The listing builds one solid part. Answer for the finished solid, in the listing's coordinates (mm). Give positions to 0.01 mm unless a question says otherwise; leave off trailing zeros. Write each loop counter-clockwise with the first axis right and the second up, starting at its lowest first coordinate (ties: lowest second). Pieces come first, ordered by that corner, then holes. Notation, with made-up numbers: M 87.5,28 L 124.5,28 A32 ccw 124.5,64 Z; hole C 39,-39.75 d10. An arc over 180 degrees is marked long. Return JSON: item names as keys, results as strings.
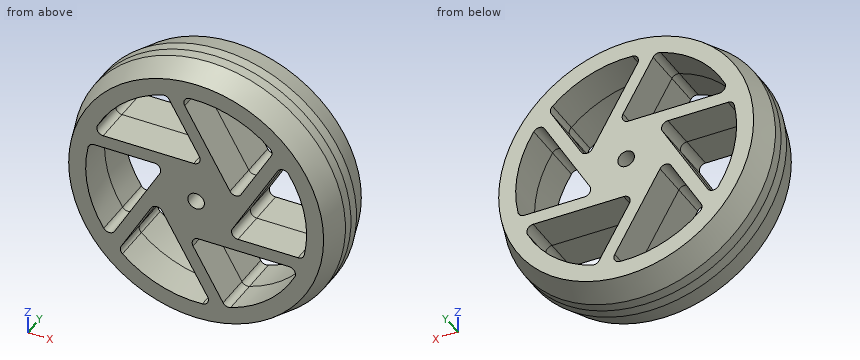
from build123d import *

# Parameters (mm, degrees)
CUT_EXTRUDE1_REACH             = 48.046
CUT_EXTRUDE1_DIRECTION_2_REACH = 48.046
CIRPATTERN1_COUNT              = 6
CUT_EXTRUDE2_DEPTH             = 15
CUT_EXTRUDE2_DEPTH_BACK        = 15
SKETCH6_R                      = 1.95


with BuildPart() as part:
    # Sketch2 → Revolve1 (revolve)
    with BuildSketch(Plane.XY, mode=Mode.PRIVATE) as revolve1_sk:
        Polygon((0, 0), (32, 0), (32, 2.5), (30, 8.5), (0, 8.5), align=None)
    revolve1 = revolve(revolve1_sk.sketch.rotate(Axis((0, 8.5, 0), (0, -1, 0)), 90), axis=Axis((0, 8.5, 0), (0, -1, 0)))

    # Mirror1: Revolve1 across plane
    add(revolve1.mirror(Plane.ZX))

    # Cut-Extrude1: up to this face of the body (flat: up to its plane)
    cut_extrude1_end = Plane(part.part.faces().sort_by_distance((0, 8.5, 0))[0])
    # Sketch3 → Cut-Extrude1 (cut, up to the picked face)
    with BuildSketch(Plane(origin=(0, 0, 0), x_dir=(1, 0, 0), z_dir=(0, 1, 0)), mode=Mode.PRIVATE) as cut_extrude1_sk1:
        with BuildLine():
            Line((0.562177826, 9.526279442), (5.5, 9.526279442))
            Line((5.5, 9.526279442), (21.878554835, 9.526279442))
            ThreePointArc((21.878554835, 9.526279442), (23.155781812, 10.23971015), (23.218058192, 11.701357775))
            ThreePointArc((23.218058192, 11.701357775), (16.957041557, 19.709356703), (8.104096566, 24.704728674))
            ThreePointArc((8.104096566, 24.704728674), (7.100974397, 24.680582577), (6.337514428, 24.029455866))
            Line((6.337514428, 24.029455866), (-0.736860279, 11.776279442))
            ThreePointArc((-0.736860279, 11.776279442), (-0.736860279, 10.276279442), (0.562177826, 9.526279442))
        make_face()
    cut_extrude1_tool1 = split(extrude(cut_extrude1_sk1.sketch, amount=CUT_EXTRUDE1_REACH, mode=Mode.PRIVATE), bisect_by=cut_extrude1_end, keep=Keep.BOTH, mode=Mode.PRIVATE)
    cut_extrude1 = cut_extrude1_tool1.solids().sort_by(Axis((10.856856, 0, -15.344995), (0, 1, 0)))[0]
    add(cut_extrude1, mode=Mode.SUBTRACT)

    # Cut-Extrude1 direction 2: up to this face of the body (flat: up to its plane)
    cut_extrude1_direction_2_end = Plane(part.part.faces().sort_by_distance((0, -8.5, 0))[0])
    # Sketch3 → Cut-Extrude1 direction 2 (cut, up to the picked face)
    with BuildSketch(Plane(origin=(0, 0, 0), x_dir=(1, 0, 0), z_dir=(0, 1, 0)), mode=Mode.PRIVATE) as cut_extrude1_direction_2_sk1:
        with BuildLine():
            Line((0.562177826, 9.526279442), (5.5, 9.526279442))
            Line((5.5, 9.526279442), (21.878554835, 9.526279442))
            ThreePointArc((21.878554835, 9.526279442), (23.155781812, 10.23971015), (23.218058192, 11.701357775))
            ThreePointArc((23.218058192, 11.701357775), (16.957041557, 19.709356703), (8.104096566, 24.704728674))
            ThreePointArc((8.104096566, 24.704728674), (7.100974397, 24.680582577), (6.337514428, 24.029455866))
            Line((6.337514428, 24.029455866), (-0.736860279, 11.776279442))
            ThreePointArc((-0.736860279, 11.776279442), (-0.736860279, 10.276279442), (0.562177826, 9.526279442))
        make_face()
    cut_extrude1_direction_2_tool1 = split(extrude(cut_extrude1_direction_2_sk1.sketch, amount=-CUT_EXTRUDE1_DIRECTION_2_REACH, mode=Mode.PRIVATE), bisect_by=cut_extrude1_direction_2_end, keep=Keep.BOTH, mode=Mode.PRIVATE)
    cut_extrude1_direction_2 = cut_extrude1_direction_2_tool1.solids().sort_by(Axis((10.856856, 0, -15.344995), (0, -1, 0)))[0]
    add(cut_extrude1_direction_2, mode=Mode.SUBTRACT)

    # CirPattern1: Cut-Extrude1, Cut-Extrude1 direction 2 ×6 about axis
    cirpattern1_axis = Axis((0, 0, 0), (0, 1, 0))
    add([cut_extrude1.rotate(cirpattern1_axis, i * 360 / CIRPATTERN1_COUNT) for i in range(1, CIRPATTERN1_COUNT)], mode=Mode.SUBTRACT)
    add([cut_extrude1_direction_2.rotate(cirpattern1_axis, i * 360 / CIRPATTERN1_COUNT) for i in range(1, CIRPATTERN1_COUNT)], mode=Mode.SUBTRACT)

    # Sketch6 → Cut-Extrude2 (cut, two sides: drawn at the far end of the back side and taken through both)
    with BuildSketch(Plane(origin=(0, 0, 0), x_dir=(1, 0, 0), z_dir=(0, 1, 0)).offset(-CUT_EXTRUDE2_DEPTH_BACK)):
        with Locations(Location((0, 0, 0), (0, 0, 270))):
            Circle(SKETCH6_R)
    extrude(amount=CUT_EXTRUDE2_DEPTH + CUT_EXTRUDE2_DEPTH_BACK, mode=Mode.SUBTRACT)


solid = part.part
Item 1: A cutting plane is placed at B-B, the plane y = 1. Count the separate pieces of the cut face and the enclosed holes in it, plus the area to 3 significant figures.
Geometry results:
{"separate pieces": "1", "enclosed holes": "7", "area": "1,740 mm2"}
Item 2: Given pin 1 Ø4 at (x, y) = (-13.5, -1) entering from +Z; pin 2 Ø10 at (x, y) = (9, 0) entering from -Z; pin 3 Ø4 at (x, y) = (-21, -6) entering from +Z; pin 4 Ø4.5 at (x, z) = (0, 0) entering from -Y, each flat-ended and moving along its own axis, determine where each tip first touches the part or whether it passes through.
Geometry results:
{"pin 1": "stops at z = 29.86", "pin 2": "stops at z = -31.75", "pin 3": "stops at z = 24.5", "pin 4": "stops at y = -8.5"}
Item 3: Find the intervals of material crossed by line 1 (X direction, y = -0.75, z = -22); line 2 (X direction, y = 0.5, z = 0); line 3 (X direction, y = -6.25, z = 14), in increasing order.
Geometry results:
{"line 1": "x = -23.24 to -13.86, 1.7 to 5.17, 13.86 to 23.24", "line 2": "x = -32 to -26, -11 to -1.95, 1.95 to 11, 26 to 32", "line 3": "x = -27.38 to -21.91, -0.55 to 2.92, 15.62 to 19.08, 21.91 to 27.38"}
Item 4: A cutting plane is placed at A-A, the plane z = 0. Write down the section's boundary in (x, y).
Geometry results:
{"outline": "M -32,-2.5 L -30,-8.5 L -26,-8.5 L -26,8.5 L -30,8.5 L -32,2.5 Z; M -11,-8.5 L -1.95,-8.5 L -1.95,8.5 L -11,8.5 Z; M 1.95,-8.5 L 11,-8.5 L 11,8.5 L 1.95,8.5 Z; M 26,-8.5 L 30,-8.5 L 32,-2.5 L 32,2.5 L 30,8.5 L 26,8.5 Z"}
